For this review, take the finished solid that the model builds, in its own axes (mm). A direction names the side the tool comes from. Round coordinates to 2 decimals unless told otherwise and drop trailing zeros. Write each loop counter-clockwise with the first axis right and the second up, starting at its lowest first coordinate (ties: lowest second). Pieces come first, ordered by that corner, then holes. Notation, with made-up numbers: (-18, 4.25) - (6, 4.25) arc R19 cw to (6, 21.25) - close; hole circle Ø6 at (10.5, 54.25). An arc over 180 degrees is marked (long way). One line per item, written item: value. Start each with the question number.
Q1. Add section D-D on y = -5.5. Write out the cut boundary in (x, z).
Q2. Clearance check with a flat-ended pin moving along its axis: pin 1 Ø3 at (y, z) = (-7.5, 2) entering from +X. State where the tip first meets the part, or that it passes through.
Q3. Add section C-C on x = 10. Write out the cut boundary in (y, z) (3 decimals).
Q4. Tool access review of faces 5 (the face through (-3, 0, 0)), 6 (the face through (8, 4.445, 3)), 7 (the face through (0, 14.605, 3)): name each direction out of +Z, -Z, +X, -X, +Y, -Y from which nothing blocks a thin tool from reaching the whole face with its end or side.
Q5. For probe 1 along X at (y, z) = (4.5, 1.95); probe 2 along Y at (x, z) = (-0.25, 3.8) (3 decimals); probe 3 along Y at (x, z) = (2.5, 1.15) (3 decimals), list the stretches that pass through material, from the lowest coordinate up.
Q6. Mouldability with a two-part tool opening along Y and no side actions: class faces 1 (the face through (8.881, -23.683, 2.576)), 2 (the face through (-2.54, 0, 3)), 3 (the face through (2.54, 9, 3)), 4 (the face through (-3, 0, 5.08)) as +Y half, -Y half, draft (parallel to the pull), parting line (faces both ways), or undercut.
Q7. Add section A-A on x = 5.75. Write out the cut boundary in (y, z) (3 decimals), and give its area (3 significant figures).
```python
from build123d import *

# Parameters (mm, degrees)
SKETCH1_W           = 25.4
SKETCH1_H           = 54.61
BOSS_EXTRUDE1_DEPTH = 5.08
FILLET1_R           = 12.7
SKETCH2_W           = 15.24
SKETCH2_H           = 19.05
CUT_EXTRUDE1_DEPTH  = 12.7
SKETCH3_W           = 5.08
SKETCH3_H           = 10.16
CUT_EXTRUDE2_DEPTH  = 12.7


with BuildPart() as part:
    # Sketch1 → Boss-Extrude1 (new body)
    with BuildSketch(Plane.XY):
        Rectangle(SKETCH1_W, SKETCH1_H)
    extrude(amount=BOSS_EXTRUDE1_DEPTH)

    # Fillet1
    fillet1_edges = [part.edges().sort_by_distance(p)[0] for p in [
        (12.7, -27.305, 2.54),
        (-12.7, -27.305, 2.54),
    ]]
    fillet(fillet1_edges, radius=FILLET1_R - 0.0001)  # a hair under: the kernel refuses the full size

    # Sketch2 → Cut-Extrude1 (cut)
    with BuildSketch(Plane.XY.offset(5.08)):
        with Locations((5.08, -5.08)):
            Rectangle(SKETCH2_W, SKETCH2_H)
    extrude(amount=-CUT_EXTRUDE1_DEPTH, mode=Mode.SUBTRACT)

    # Sketch3 → Cut-Extrude2 (cut)
    with BuildSketch(Plane.XY.offset(5.08)):
        with Locations((0, 9.525)):
            Rectangle(SKETCH3_W, SKETCH3_H)
    extrude(amount=-CUT_EXTRUDE2_DEPTH, mode=Mode.SUBTRACT)


solid = part.part
```
Result set:
1. outline: (-12.7, 0) - (-2.54, 0) - (-2.54, 5.08) - (-12.7, 5.08) - close
2. pin 1: stops at x = -2.54
3. outline: (-22.434, 0) - (-14.605, 0) - (-14.605, 5.08) - (-22.434, 5.08) - close; (4.445, 0) - (27.305, 0) - (27.305, 5.08) - (4.445, 5.08) - close
4. face 5: -Z, +X, -X, +Y, -Y
4. face 6: +Z, -Z, +X
4. face 7: +Z, -Z
5. probe 1: x = -12.7 to -2.54, 2.54 to 12.7
5. probe 2: y = -27.303 to -14.605, 14.605 to 27.305
5. probe 3: y = -27.057 to -14.605, 14.605 to 27.305
6. face 1: -Y half
6. face 2: undercut
6. face 3: undercut
6. face 4: draft
7. outline: (-25.929, 0) - (-14.605, 0) - (-14.605, 5.08) - (-25.929, 5.08) - close; (4.445, 0) - (27.305, 0) - (27.305, 5.08) - (4.445, 5.08) - close
7. area: 174 mm^2
